from build123d import *


with BuildPart() as f1:
    # F0 (on Top) → F1 (revolve)
    with BuildSketch(Plane.XY):
        with BuildLine():
            Line((11.458813, 46.930371), (-0.244609, 67.031535))
            Line((-0.244609, 67.031535), (-0.244609, 20.647742))
            Line((-0.244609, 20.647742), (4.516693, 20.647742))
            Line((4.516693, 20.647742), (4.516693, -20.192879))
            Line((4.516693, -20.192879), (12.459272, -20.192879))
            Line((12.459272, -20.192879), (12.459272, -4.814634))
            Line((12.459272, -4.814634), (27.12154, -4.814634))
            Line((27.12154, -4.814634), (36.102078, 4.604435))
            Line((36.102078, 4.604435), (7.908328, 4.604435))
            Line((7.908328, 4.604435), (28.964354, 16.863803))
            Line((28.964354, 16.863803), (14.195322, 20.647742))
            ThreePointArc((14.195322, 20.647742), (3.67909, 32.836583), (11.458813, 46.930371))
        make_face()
        with BuildLine():
            Line((12.459272, -20.192879), (4.516693, -20.192879))
            Line((4.516693, -20.192879), (0, -20.192879))
            Line((0, -20.192879), (0, -28.713265))
            Line((0, -28.713265), (31.294234, -28.713265))
            ThreePointArc((31.294234, -28.713265), (22.795528, -22.422049), (12.459272, -20.192879))
        make_face()
    revolve(axis=Axis((-0.244609, 43.839638, 0), (0, -1, 0)))


solid = f1.part
Work out the finished part from the listing and answer in its coordinate system (mm). A direction names the side the tool comes from. Coordinates: 2 decimals unless noted, no trailing zeros. Write each loop counter-clockwise with the first axis right and the second up, starting at its lowest first coordinate (ties: lowest second). Pieces come first, ordered by that corner, then holes.
1. The part is cut by section D-D, the plane y = 56. Write down the section's boundary in (x, z), and give its area (3 significant figures).
Results list:
outline: circle Ø12.85 at (-0.24, 0)
area: 130 mm2
2. Consider line 1 along Y through (x, z) = (-20, -16); line 2 along Y through (x, z) = (-15, -3.5); line 3 along Y through (x, z) = (-1.5, -31). Determine where each line is inside the solid, lowest interval first.
Results list:
line 1: y = -28.71 to -23.66, -4.81 to 4.6, 14.66 to 17.83
line 2: y = -28.71 to -20.31, -4.81 to 4.6, 8.69 to 20.46
line 3: y = -28.71 to -28.15, -0.98 to 4.6
3. Flat-ended cylindrical pins translate along their axes: pin 1 (5 mm diameter, centred on x = -0.5, z = -1.5, fed in from +Y); pin 2 (1 mm diameter, centred on y = 1, z = -9, fed in from +X); pin 3 (22 mm diameter, centred on x = 7, z = -9.5, fed in from +Y); pin 4 (10 mm diameter, centred on x = -26.5, y = 21, fed in from +Z). Find the tip coordinate at first contact, or state that the pin passes through.
Results list:
pin 1: stops at y = 67.03
pin 2: stops at x = 31.93
pin 3: stops at y = 65.4
pin 4: stops at z = 17.42
4. The part is cut by section B-B, the plane y = -1.5. Write down the section's boundary in (x, z).
Results list:
outline: circle Ø61.05 at (-0.24, 0); hole circle Ø9.52 at (-0.24, 0)
5. For faces 1 (the flat face through (0.2, -28.713, 0.4)), 2 (the conical face through (-6.3, -4.23, -27.26)), determine the directions among +Z, -Z, +X, -X, +Y, -Y from which every point of the face is accessible in a straight line to the end or side of a thin tool.
Results list:
face 1: +Z, -Z, +X, -X, -Y
face 2: none
6. The part is cut by section A-A, the plane x = -9.5. State how many separate pieces and enclosed holes the cut face has, and give its area (3 significant figures).
Results list:
separate pieces: 3
enclosed holes: 0
area: 1,860 mm2
7. For a pull along Z with two mould halves and no side action, classify faces 3 (the cylindrical face through (-1.898, -12.396, 12.596)), 4 (the flat face through (0, 20.648, 0)), 5 (the flat face through (-6, -4.815, -12)) as +Z half, -Z half, draft (parallel to the pull), parting line (faces both ways), or undercut.
Results list:
face 3: parting line
face 4: undercut
face 5: draft
